from build123d import *

# Parameters (mm, degrees)
IZIM1_W                     = 63
IZIM1_H                     = 80
Y_KSEKLIK_EKSTR_ZYON1_DEPTH = 1.5
IZIM2_R                     = 1
KES_EKSTR_ZYON1_DEPTH       = 1.5
RADYUS1_R                   = 2
PAH1_SIZE                   = 0.5


with BuildPart() as part:
    # Çizim1 → Yükseklik-Ekstrüzyon1 (new body)
    with BuildSketch(Plane.XY):
        Rectangle(IZIM1_W, IZIM1_H)
    extrude(amount=Y_KSEKLIK_EKSTR_ZYON1_DEPTH)

    # Çizim2 → Kes-Ekstrüzyon1 (cut)
    with BuildSketch(Plane.XY.offset(1.5)):
        with Locations((-29.25, 37.75)):
            Circle(IZIM2_R)
        with Locations(Location((29.25, 37.75, 0), (0, 0, 180))):
            Circle(IZIM2_R)
        with Locations((29.25, -37.75)):
            Circle(IZIM2_R)
        with Locations(Location((-29.25, -37.75, 0), (0, 0, 180))):
            Circle(IZIM2_R)
    extrude(amount=-KES_EKSTR_ZYON1_DEPTH, mode=Mode.SUBTRACT)

    # Radyus1
    radyus1_edges = [part.edges().sort_by_distance(p)[0] for p in [
        (31.5, -40, 0.75),
        (-31.5, -40, 0.75),
        (-31.5, 40, 0.75),
        (31.5, 40, 0.75),
    ]]
    fillet(radyus1_edges, radius=RADYUS1_R)

    # Pah1
    pah1_edges = [part.edges().sort_by_distance(p)[0] for p in [
        (-28.25, -37.75, 1.5),
        (28.25, -37.75, 1.5),
        (30.25, 37.75, 1.5),
        (-30.25, 37.75, 1.5),
    ]]
    chamfer(pah1_edges, length=PAH1_SIZE)


solid = part.part
Check sheet for the modelled part. Datum: model origin and axes. Units: mm. Give positions to 0.01 mm unless a question says otherwise; leave off trailing zeros. Return JSON: item names as keys, results as strings. Group by question number.
1. Go/stop test with flat-tipped pins: pin 1 (2.5 mm diameter, centred on x = 29.25, y = 37.75, fed in from +Z); pin 2 (1.2 mm diameter, centred on x = -29.25, y = 37.75, fed in from +Z); pin 3 (1 mm diameter, centred on x = -19.5, y = -16, fed in from -Z). Record where each tip stops, or that it passes through.
2. Thickness scan on L1, parallel to Y at x = -29.25, z = 0.5. Record the ranges inside material, lowest first.
3. Mould release check, pull along Y, two halves, no side actions. Record for faces 1 (the cylindrical face through (30.9, -39.43, 0.76)), 2 (the flat face through (0, 1, 0)), 3 (the cylindrical face through (-28.71, 38.59, 0.51)): released by +Y, released by -Y, zero draft, split by the parting line, or undercut.
Return value:
{
 "1": {"pin 1": "z = 1.25", "pin 2": "through", "pin 3": "z = 0"},
 "2": {"L1": "-40 to -38.75, -36.75 to 36.75, 38.75 to 40"},
 "3": {"face 1": "released by -Y", "face 2": "zero draft", "face 3": "undercut"}
}
